Source: CAD feature listing. Evaluate the final solid. Frame: model axes, mm. Face numbers are marked on the shaded views. A direction names the side the tool comes from. Give positions to 0.01 mm unless a question says otherwise; leave off trailing zeros. Answer in a Markdown table with one row per item.
```python
from build123d import *

# Parameters (mm, degrees)
F0_W     = 12.7
F0_H     = 12.7
F0_R     = 1.5875
F1_DEPTH = 6.35
F2_DEPTH = 25.4
F3_R     = 1.5875
F4_DEPTH = 25.4
F5_R     = 1.27
F6_SIZE  = 0.3175


with BuildPart() as f1:
    # F0 (on Top) → F1 (new body)
    with BuildSketch(Plane.XY):
        with Locations((0, 12.7)):
            Rectangle(F0_W, F0_H)
        with Locations((0, 12.7)):
            Circle(F0_R, mode=Mode.SUBTRACT)
    extrude(amount=F1_DEPTH)



with BuildPart() as f1b:
    # F0 (on Top) → F1, piece 2 (new body)
    with BuildSketch(Plane.XY):
        with Locations((0, -12.7)):
            Rectangle(F0_W, F0_H)
        with Locations((0, -12.7)):
            Circle(F0_R, mode=Mode.SUBTRACT)
    extrude(amount=F1_DEPTH)


with BuildPart() as f1_1:
    add(f1.part)

    add(f1b.part)  # F2 merges F1b
    # F0 (on Top) → F2 (join)
    with BuildSketch(Plane.XY):
        Rectangle(F0_W, F0_H)
    extrude(amount=F2_DEPTH)

    # F3 (on face) → F4 (cut)
    with BuildSketch(Plane(origin=(0, 6.35, 0), x_dir=(-1, 0, 0), z_dir=(0, 1, 0))):
        with Locations((0, 19.05)):
            Circle(F3_R)
    extrude(amount=-F4_DEPTH, mode=Mode.SUBTRACT)

    # F5
    f5_edges = [f1_1.edges().sort_by_distance(p)[0] for p in [
        (0, 6.35, 25.4),
        (6.35, 0, 25.4),
        (0, -6.35, 25.4),
        (-6.35, 0, 25.4),
        (6.35, 6.35, 15.875),
        (6.35, -6.35, 15.875),
        (6.35, -12.7, 6.35),
        (6.35, 12.7, 6.35),
        (-6.35, 6.35, 15.875),
        (-6.35, 12.7, 6.35),
        (-6.35, -6.35, 15.875),
        (-6.35, -12.7, 6.35),
        (0, -19.05, 6.35),
        (-6.35, -19.05, 3.175),
        (6.35, -19.05, 3.175),
        (6.35, 19.05, 3.175),
        (-6.35, 19.05, 3.175),
        (0, 19.05, 6.35),
    ]]
    fillet(f5_edges, radius=F5_R)

    # F6
    f6_edges = [f1_1.edges().sort_by_distance(p)[0] for p in [
        (-1.5875, -12.7, 6.35),
        (-1.5875, 12.7, 6.35),
        (1.5875, 6.35, 19.05),
        (1.5875, -6.35, 19.05),
    ]]
    chamfer(f6_edges, length=F6_SIZE)


solid = f1_1.part
```
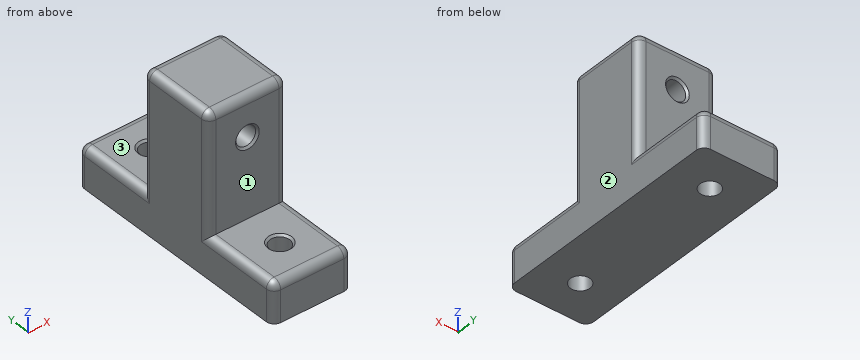
Q1. Reachability of the marked faces 1, 2 and 3 from +Z, -Z, +X, -X, +Y, -Y: full face, straight path, thin tool, end or side. Return the list, or none.
Values follow:
| item | result |
|---|---|
| face 1 | +Z, +X, -X, -Y |
| face 2 | +Z, -Z, +X, +Y, -Y |
| face 3 | +Z, +X, -X, +Y |
Q2. Ray query, probe 1 along Y at (x, z) = (0, 4); probe 2 along Z at (x, y) = (0, -0.5); probe 3 along Z at (x, y) = (4.25, 11.5). Return the intervals inside material, ascending. Write a range as from..to.
Values follow:
| item | result |
|---|---|
| probe 1 | -19.05..-14.29, -11.11..11.11, 14.29..19.05 |
| probe 2 | 0..17.46, 20.64..25.4 |
| probe 3 | 0..6.35 |
Q3. Section query C-C (x = 0). Give the number of separate pieces and of enclosed holes in the cut face, plus the area to 3 significant figures.
Values follow:
| item | result |
|---|---|
| separate pieces | 4 |
| enclosed holes | 0 |
| area | 401 mm^2 |
Q4. Contact query for flat-ended pins moving along their axis: pin 1 Ø5 at (x, y) = (-1, 11) entering from +Z; pin 2 Ø3 at (x, z) = (-1, 14.5) entering from -Y; pin 3 Ø1.5 at (x, y) = (-5, 9.5) entering from -Z; pin 4 Ø1.5 at (x, z) = (0.5, 20.5) entering from +Y. Output: stop coordinate, or through.
Values follow:
| item | result |
|---|---|
| pin 1 | z = 6.35 |
| pin 2 | y = -6.35 |
| pin 3 | z = 0 |
| pin 4 | y = 6.35 |
